Check sheet for the drawn part. Datum: minimum x, y, z corner. Units: mm. A direction names the side the tool comes from. Round coordinates to 2 decimals unless told otherwise and drop trailing zeros. Order: outer loops, then holes, each group sorted by start corner. A loop starts at its lowest first (then second) coordinate and runs counter-clockwise, first axis right, second up. Notation, with made-up numbers: M -11.5,-21.75 L -6.5,-21.75 A8 cw -6.5,-17.75 Z; hole C -11,70.25 d7. An arc over 180 degrees is marked long. Use one line per item in the form item = value. Start each with the question number.
Item 1: Go/stop test with flat-tipped pins: pin 1 Ø16 at (x, y) = (10, 10) entering from +Z; pin 2 Ø4 at (x, z) = (16.5, 17) entering from +Y; pin 3 Ø5 at (x, z) = (23, 16) entering from -Y. Record where each tip stops, or that it passes through.
Item 2: Cross-section at D-D on y = 35. Enter the section's corners in (x, z).
Item 3: Cross-section at A-A on y = 8. Enter the section's corners in (x, z).
Item 4: Thickness scan on probe 1 along Y at (x, z) = (50, 7.25); probe 2 along X at (y, z) = (54.5, 8.75); probe 3 along Z at (x, y) = (23.5, 6.5). Record the ranges inside material, lowest first. Write a range as [from, to].
Item 5: Cross-section at B-B on z = 8. Enter the section's corners in (x, y).
Item 6: Tool access check on the marked faces 1 and 2. Record the directions out of +Z, -Z, +X, -X, +Y, -Y that give a thin tool (end or side, any length) a straight path to the whole face; none if there is none.
Item 7: Release check for a two-part mould opening along X. For the marked faces 3, 4 and 5 record: +X half, -X half, draft (parallel to the pull), parting line (faces both ways), or undercut.
Item 8: Cross-section at C-C on x = 32.5. Enter the section's corners in (y, z), then the cut area to 3 significant figures.
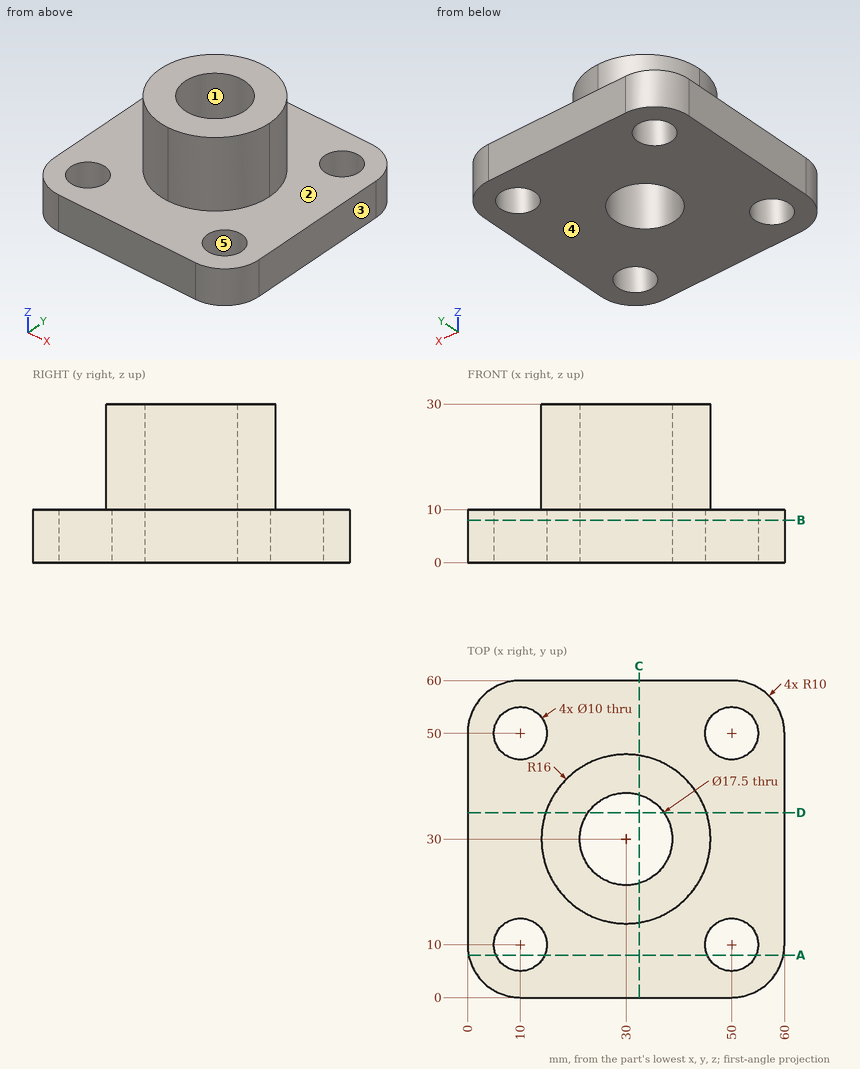
Output values:
q1.pin_1 = 10
q1.pin_2 = 41.12
q1.pin_3 = 14.65
q2.outline = M 0,0 L 22.82,0 L 22.82,30 L 14.8,30 L 14.8,10 L 0,10 Z; M 37.18,0 L 60,0 L 60,10 L 45.2,10 L 45.2,30 L 37.18,30 Z
q3.outline = M 0.2,0 L 5.42,0 L 5.42,10 L 0.2,10 Z; M 14.58,0 L 45.42,0 L 45.42,10 L 14.58,10 Z; M 54.58,0 L 59.8,0 L 59.8,10 L 54.58,10 Z
q4.probe_1 = [0, 5], [15, 45], [55, 60]
q4.probe_2 = [1.07, 7.82], [12.18, 47.82], [52.18, 58.93]
q4.probe_3 = [0, 10]
q5.outline = M 0,10 A10 ccw 10,0 L 50,0 A10 ccw 60,10 L 60,50 A10 ccw 50,60 L 10,60 A10 ccw 0,50 Z; hole C 10,10 d10; hole C 10,50 d10; hole C 30,30 d17.5; hole C 50,10 d10; hole C 50,50 d10
q6.face_1 = +Z, -Z
q6.face_2 = +Z
q7.face_3 = +X half
q7.face_4 = draft
q7.face_5 = undercut
q8.outline = M 0,0 L 21.61,0 L 21.61,30 L 14.2,30 L 14.2,10 L 0,10 Z; M 38.39,0 L 60,0 L 60,10 L 45.8,10 L 45.8,30 L 38.39,30 Z
q8.area = 729 mm2
